Geometry: final body of the model. Coordinates: model frame, mm. A direction names the side the tool comes from. Round coordinates to 2 decimals unless told otherwise and drop trailing zeros. Order: outer loops, then holes, each group sorted by start corner. A loop starts at its lowest first (then second) coordinate and runs counter-clockwise, first axis right, second up. Notation, with made-up numbers: (7, -8.75) - (55, -8.75) arc R29 cw to (55, 23.25) - close; hole circle Ø2 at (71.25, 32.25). An arc over 180 degrees is marked (long way). Put each result on its own line as item: value. Start each with the question number.
(1) Pull-direction query (Y, two-part tool) for faces 1 (the face through (-15, 12.75, 11)), 2 (the face through (-15, -7.75, 11)), 3 (the face through (18.3, -16, 21)), 4 (the face through (-10.33, -12.68, 8.52)); classes: released by +Y, released by -Y, zero draft, split by the parting line, or undercut.
(2) Material intervals for L1, parallel to X at y = -8.5, z = 10.25; L2, parallel to Y at x = 0, z = 16.75; L3, parallel to Z at x = -12, y = 13, sorted ascending. Write a range as [from, to].
(3) Access query for faces 5 (the face through (-15, -1.25, 11)), 6 (the face through (-10.272, -12.68, 15.448)), 7 (the face through (56.7, 0, 18)). Directions: +Z, -Z, +X, -X, +Y, -Y. A direction counts if a zero-diameter tool reaches every point of the face in a straight line with its end or side. Return the directions, or none.
(4) Pin query (flat end, axial travel): P1, Ø7.5, axis at x = 19.2, y = 12, coming from the +Z side; P2, Ø8.5, axis at x = 19.2, y = -12, coming from the -Z side; P3, Ø10, axis at y = -12.5, z = 4, coming from the +X side. Return the tip coordinate at first contact, or that it passes through.
(5) Section C-C (z = 12). Output: boundary loops of the cut face in (x, y).
(6) Section A-A (y = 12). Output: boundary loops of the cut face in (x, z), and give its area (3 significant figures).
(7) Section D-D (y = -12). Output: boundary loops of the cut face in (x, z).
(8) Section B-B (x = 19.2). Output: boundary loops of the cut face in (y, z), and give its area (3 significant figures).
from build123d import *

# Parameters (mm, degrees)
ESQUISSE1_R             = 2.1
BOSS_EXTRU_1_DEPTH      = 22
ESQUISSE2_W             = 52.543778308
ESQUISSE2_H             = 17.447246457
ENL_V_MAT_EXTRU_1_DEPTH = 42
ESQUISSE3_R             = 3.1
ESQUISSE3_R_2           = 3.6
ENL_V_MAT_EXTRU_2_DEPTH = 2
D_GAGEMENT_M51_D        = 5.3
D_GAGEMENT_M51_DEPTH    = 34
D_GAGEMENT_M51_TIP      = 1.59228064
ESQUISSE6_R             = 4
ENL_V_MAT_EXTRU_3_DEPTH = 3
ENL_V_MAT_EXTRU_4_DEPTH = 8
ESQUISSE8_R             = 1.25
ENL_V_MAT_EXTRU_5_DEPTH = 5
BOSS_EXTRU_2_START      = 2
ESQUISSE9_R             = 4
BOSS_EXTRU_2_DEPTH      = 2
BOSS_EXTRU_3_DEPTH      = 2
ESQUISSE11_R            = 2.6
ENL_V_MAT_EXTRU_6_DEPTH = 10
ESQUISSE12_R            = 4.1
ENL_V_MAT_EXTRU_7_DEPTH = 2


with BuildPart() as part:
    # Esquisse1 → Boss.-Extru.1 (new body)
    with BuildSketch(Plane.XY):
        with BuildLine():
            Line((-18.3, 1.25), (-7.901740315, 1.25))
            ThreePointArc((-7.901740315, 1.25), (8, 0), (-7.901740315, -1.25))
            Line((-7.901740315, -1.25), (-18.3, -1.25))
            Line((-18.3, -1.25), (-18.3, -15.75))
            Line((-18.3, -15.75), (61.7, -15.75))
            Line((61.7, -15.75), (61.7, 15.75))
            Line((61.7, 15.75), (-18.3, 15.75))
            Line((-18.3, 15.75), (-18.3, 1.25))
        make_face()
        with Locations((19.2, -12)):
            Circle(ESQUISSE1_R, mode=Mode.SUBTRACT)
        with Locations((54.2, -12)):
            Circle(ESQUISSE1_R, mode=Mode.SUBTRACT)
        with Locations((54.2, 12)):
            Circle(ESQUISSE1_R, mode=Mode.SUBTRACT)
        with Locations((19.2, 12)):
            Circle(ESQUISSE1_R, mode=Mode.SUBTRACT)
    extrude(amount=BOSS_EXTRU_1_DEPTH)

    # Esquisse2 → Enlèv. mat.-Extru.1 (cut)
    with BuildSketch(Plane(origin=(0, 15.75, 0), x_dir=(1, 0, 0), z_dir=(0, 1, 0))):
        with Locations((37.971889154, -5.276376771)):
            Rectangle(ESQUISSE2_W, ESQUISSE2_H)
    extrude(amount=-ENL_V_MAT_EXTRU_1_DEPTH, mode=Mode.SUBTRACT)

    # Esquisse3 → Enlèv. mat.-Extru.2 (cut)
    with BuildSketch(Plane.XY.offset(22)):
        with Locations((19.2, -12)):
            Circle(ESQUISSE3_R)
        with Locations((54.2, -12)):
            Circle(ESQUISSE3_R)
        with Locations((54.2, 12)):
            Circle(ESQUISSE3_R_2)
        with Locations((19.2, 12)):
            Circle(ESQUISSE3_R)
    extrude(amount=-ENL_V_MAT_EXTRU_2_DEPTH, mode=Mode.SUBTRACT)

    # Dégagement M51
    with Locations(Plane(origin=(0, 15.75, 0), x_dir=(1, 0, 0), z_dir=(0, 1, 0))):
        with Locations((-12.3, -12)):
            Hole(D_GAGEMENT_M51_D / 2, depth=D_GAGEMENT_M51_DEPTH)
            with Locations((0, 0, -(D_GAGEMENT_M51_DEPTH + D_GAGEMENT_M51_TIP / 2))):  # 118° drill point
                Cone(0, D_GAGEMENT_M51_D / 2, D_GAGEMENT_M51_TIP, mode=Mode.SUBTRACT)

    # Esquisse6 → Enlèv. mat.-Extru.3 (cut)
    with BuildSketch(Plane(origin=(0, 15.75, 0), x_dir=(1, 0, 0), z_dir=(0, 1, 0))):
        with Locations(Location((-12.3, -12, 0), (0, 0, 180))):
            Circle(ESQUISSE6_R)
    extrude(amount=-ENL_V_MAT_EXTRU_3_DEPTH, mode=Mode.SUBTRACT)

    # Esquisse7 → Enlèv. mat.-Extru.4 (cut)
    with BuildSketch(Plane.XZ.offset(15.75)):
        Polygon((-12.3, 16.618802154), (-16.3, 14.309401077), (-16.3, 9.690598923), (-12.3, 7.381197846), (-8.3, 9.690598923), (-8.3, 14.309401077), align=None)
    extrude(amount=-ENL_V_MAT_EXTRU_4_DEPTH, mode=Mode.SUBTRACT)

    # Esquisse8 → Enlèv. mat.-Extru.5 (cut)
    with BuildSketch(Plane(origin=(61.7, 0, 0), x_dir=(0, 0, -1), z_dir=(1, 0, 0))):
        with Locations(Location((-18, 0, 0), (0, 0, 90))):
            Circle(ESQUISSE8_R)
    extrude(amount=-ENL_V_MAT_EXTRU_5_DEPTH, mode=Mode.SUBTRACT)

    # Esquisse9 → Boss.-Extru.2 (add)
    with BuildSketch(Plane(origin=(0, 15.75, 0), x_dir=(1, 0, 0), z_dir=(0, 1, 0)).offset(BOSS_EXTRU_2_START)):
        Polygon((61.7, -22), (61.7, -14), (11.7, -14), (11.7, 0), (-18.3, 0), (-18.3, -22), align=None)
        with Locations(Location((-12.3, -12, 0), (0, 0, 180))):
            Circle(ESQUISSE9_R, mode=Mode.SUBTRACT)
    extrude(amount=-BOSS_EXTRU_2_DEPTH)

    # Esquisse10 → Boss.-Extru.3 (add)
    with BuildSketch(Plane.XZ.offset(15.75)):
        Polygon((11.7, 0), (11.7, 14), (61.7, 14), (61.7, 22), (-18.3, 22), (-18.3, 0), align=None)
        Polygon((-12.3, 16.618802154), (-16.3, 14.309401077), (-16.3, 9.690598923), (-12.3, 7.381197846), (-8.3, 9.690598923), (-8.3, 14.309401077), align=None, mode=Mode.SUBTRACT)
    extrude(amount=BOSS_EXTRU_3_DEPTH)

    # Esquisse11 → Enlèv. mat.-Extru.6 (cut)
    with BuildSketch(Plane.XY.offset(20)):
        with Locations((54.2, 12)):
            Circle(ESQUISSE11_R)
        with Locations((54.2, -12)):
            Circle(ESQUISSE11_R)
        with Locations((19.2, -12)):
            Circle(ESQUISSE11_R)
        with Locations((19.2, 12)):
            Circle(ESQUISSE11_R)
    extrude(amount=-ENL_V_MAT_EXTRU_6_DEPTH, mode=Mode.SUBTRACT)

    # Esquisse12 → Enlèv. mat.-Extru.7 (cut)
    with BuildSketch(Plane.XY.offset(22)):
        with Locations((54.2, -12)):
            Circle(ESQUISSE12_R)
        with Locations((19.2, -12)):
            Circle(ESQUISSE12_R)
        with Locations((19.2, 12)):
            Circle(ESQUISSE12_R)
        with Locations((54.2, 12)):
            Circle(ESQUISSE12_R)
    extrude(amount=-ENL_V_MAT_EXTRU_7_DEPTH, mode=Mode.SUBTRACT)


solid = part.part
Checks:
1. face 1: released by +Y
1. face 2: released by -Y
1. face 3: undercut
1. face 4: zero draft
2. L1: x = [-18.3, -16.3], [-8.3, 11.7]
2. L2: y = [-17.75, -8], [8, 17.75]
2. L3: z = [0, 8.01], [15.99, 22]
3. face 5: +Z, -Z, -X
3. face 6: -Y
3. face 7: +X
4. P1: stops at z = 20
4. P2: stops at z = 14
4. P3: stops at x = 11.7
5. outline: (-18.3, -17.75) - (-16.3, -17.75) - (-16.3, -7.75) - (-14.95, -7.75) - (-14.95, -1.25) - (-18.3, -1.25) - close; (-18.3, 1.25) - (-14.95, 1.25) - (-14.95, 12.75) - (-16.3, 12.75) - (-16.3, 17.75) - (-18.3, 17.75) - close; (-9.65, -7.75) - (-8.3, -7.75) - (-8.3, -17.75) - (11.7, -17.75) - (11.7, 17.75) - (-8.3, 17.75) - (-8.3, 12.75) - (-9.65, 12.75) - (-9.65, 1.25) - (-7.9, 1.25) arc R8 cw (long way) to (-7.9, -1.25) - (-9.65, -1.25) - close
6. outline: (-18.3, 0) - (11.7, 0) - (11.7, 14) - (16.6, 14) - (16.6, 20) - (15.1, 20) - (15.1, 22) - (-18.3, 22) - close; (21.8, 14) - (51.6, 14) - (51.6, 20) - (50.1, 20) - (50.1, 22) - (23.3, 22) - (23.3, 20) - (21.8, 20) - close; (56.8, 14) - (61.7, 14) - (61.7, 22) - (58.3, 22) - (58.3, 20) - (56.8, 20) - close; hole circle Ø5.3 at (-12.3, 12)
6. area: 943 mm²
7. outline: (-18.3, 0) - (11.7, 0) - (11.7, 14) - (16.6, 14) - (16.6, 20) - (15.1, 20) - (15.1, 22) - (-18.3, 22) - close; (21.8, 14) - (51.6, 14) - (51.6, 20) - (50.1, 20) - (50.1, 22) - (23.3, 22) - (23.3, 20) - (21.8, 20) - close; (56.8, 14) - (61.7, 14) - (61.7, 22) - (58.3, 22) - (58.3, 20) - (56.8, 20) - close; hole (-16.3, 9.69) - (-12.3, 7.38) - (-8.3, 9.69) - (-8.3, 14.31) - (-12.3, 16.62) - (-16.3, 14.31) - close
8. outline: (-17.75, 14) - (-14.6, 14) - (-14.6, 20) - (-16.1, 20) - (-16.1, 22) - (-17.75, 22) - close; (-9.4, 14) - (9.4, 14) - (9.4, 20) - (7.9, 20) - (7.9, 22) - (-7.9, 22) - (-7.9, 20) - (-9.4, 20) - close; (14.6, 14) - (17.75, 14) - (17.75, 22) - (16.1, 22) - (16.1, 20) - (14.6, 20) - close
8. area: 189 mm²
